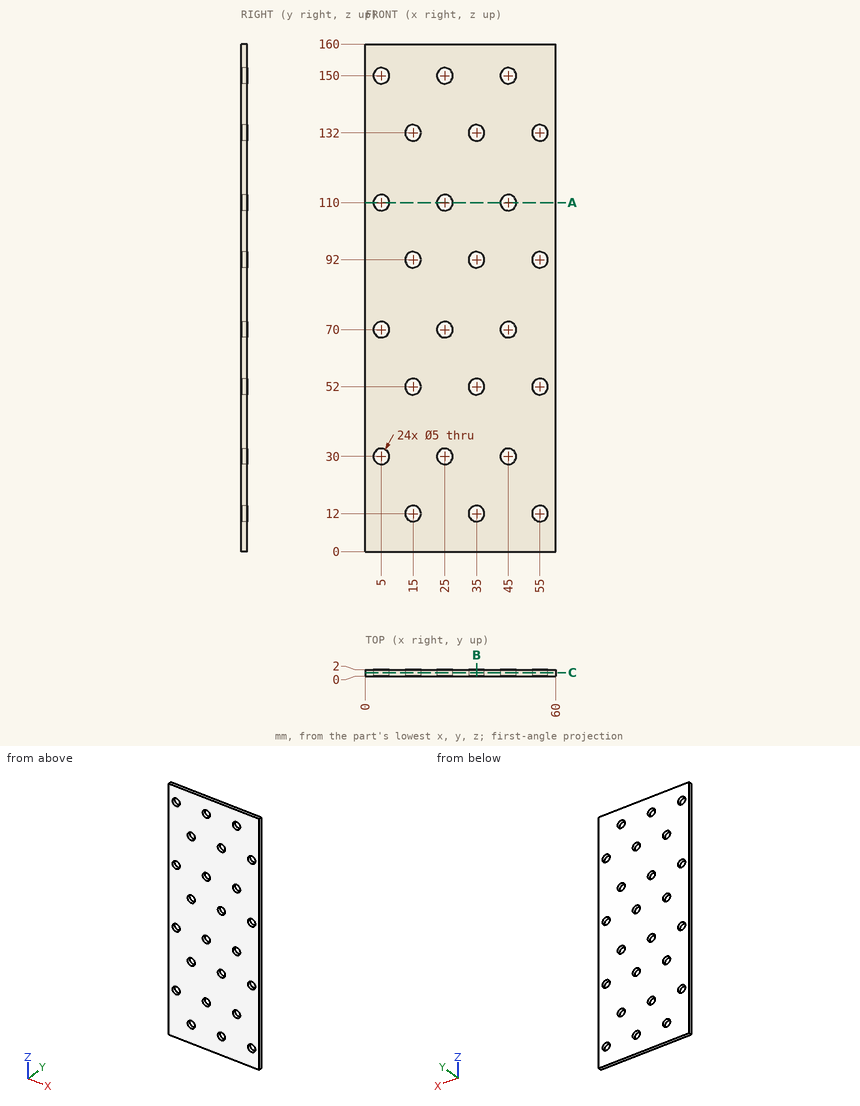
Could you check a few things on this drawing? It's one solid part, dimensions in mm from its lowest x, y, z. Round coordinates to 2 decimals unless told otherwise and drop trailing zeros. Order: outer loops, then holes, each group sorted by start corner. A loop starts at its lowest first (then second) coordinate and runs counter-clockwise, first axis right, second up.
Q1. Imagine slicing it at B-B, the plane x = 35. List the corners of the cut face in (y, z) for me.
Geometry says:
outline: (0, 0) - (2, 0) - (2, 9.5) - (0, 9.5) - close; (0, 14.5) - (2, 14.5) - (2, 49.5) - (0, 49.5) - close; (0, 54.5) - (2, 54.5) - (2, 89.5) - (0, 89.5) - close; (0, 94.5) - (2, 94.5) - (2, 129.5) - (0, 129.5) - close; (0, 134.5) - (2, 134.5) - (2, 160) - (0, 160) - close
Q2. Imagine slicing it at A-A, the plane z = 110. List the corners of the cut face in (x, y) for me.
Geometry says:
outline: (0, 0) - (2.5, 0) - (2.5, 2) - (0, 2) - close; (7.5, 0) - (22.5, 0) - (22.5, 2) - (7.5, 2) - close; (27.5, 0) - (42.5, 0) - (42.5, 2) - (27.5, 2) - close; (47.5, 0) - (60, 0) - (60, 2) - (47.5, 2) - close
Q3. Imagine slicing it at C-C, the plane y = 1.05. State how many separate pieces and enclosed holes the cut face has, then the cut area to 3 significant figures.
Geometry says:
separate pieces: 1
enclosed holes: 24
area: 9,130 mm2
Q4. Please list where these lines run through material, in increasing order: probe 1 along Z at (x, y) = (45, 1.4); probe 2 along Z at (x, y) = (15, 0.95); probe 3 along X at (y, z) = (0.2, 132).
Geometry says:
probe 1: z = 0 to 27.5, 32.5 to 67.5, 72.5 to 107.5, 112.5 to 147.5, 152.5 to 160
probe 2: z = 0 to 9.5, 14.5 to 49.5, 54.5 to 89.5, 94.5 to 129.5, 134.5 to 160
probe 3: x = 0 to 12.5, 17.5 to 32.5, 37.5 to 52.5, 57.5 to 60
Q5. I'm going to push a flat-ended pin straight in: P1, Ø4.5, axis at x = 5, z = 110, coming from the +Y side. Where does the tip first touch, or does it pass through?
Geometry says:
P1: passes through
